from build123d import *

# Parameters (mm, degrees)
SKETCH2_R           = 1.5
BOSS_EXTRUDE1_DEPTH = 5


with BuildPart() as part:
    # Sketch2 → Boss-Extrude1 (new body)
    with BuildSketch(Plane.XY):
        with BuildLine():
            Line((5, -33), (5, -8.660254038))
            ThreePointArc((5, -8.660254038), (9.870667346, 1.603098918), (2.002269745, 9.797495388))
            Line((2.002269745, 9.797495388), (2.00266405, 11.49953636))
            Line((2.00266405, 11.49953636), (2.002664157, 11.499999691))
            ThreePointArc((2.002664157, 11.499999691), (0.002664157, 13.499999691), (-1.997335843, 11.499999691))
            Line((-1.997335843, 11.499999691), (-1.998003665, 8.617307095))
            ThreePointArc((-1.998003665, 8.617307095), (-3.567262635, 6.664705601), (-5.812270881, 7.776085051))
            Line((-5.812270881, 7.776085051), (-6.351761581, 8.938967191))
            ThreePointArc((-6.351761581, 8.938967191), (-9.315039529, 9.734283484), (-9.574251776, 6.677102885))
            Line((-9.574251776, 6.677102885), (-7.526953052, 4.647039677))
            ThreePointArc((-7.526953052, 4.647039677), (-7.244787999, 2.157941439), (-9.614515081, 1.345771067))
            Line((-9.614515081, 1.345771067), (-10.820227093, 1.781203427))
            ThreePointArc((-10.820227093, 1.781203427), (-13.469614339, 0.244947506), (-11.499566198, -2.099886252))
            Line((-11.499566198, -2.099886252), (-11.463831285, -2.099566981))
            Line((-11.463831285, -2.099566981), (-8.600020221, -2.073980428))
            ThreePointArc((-8.600020221, -2.073980428), (-6.633040893, -3.625608638), (-7.724488765, -5.880669462))
            Line((-7.724488765, -5.880669462), (-7.993660259, -6.008443697))
            Line((-7.993660259, -6.008443697), (-8.882563754, -6.430401321))
            ThreePointArc((-8.882563754, -6.430401321), (-9.651698384, -9.400582629), (-6.592349134, -9.632805038))
            Line((-6.592349134, -9.632805038), (-5.601479532, -8.615725566))
            ThreePointArc((-5.601479532, -8.615725566), (-5.218458324, -8.535632344), (-5, -8.860280046))
            Line((-5, -8.860280046), (-5, -33))
            ThreePointArc((-5, -33), (0, -38), (5, -33))
        make_face()
        with Locations((0, -33)):
            Circle(SKETCH2_R, mode=Mode.SUBTRACT)
        Circle(SKETCH2_R, mode=Mode.SUBTRACT)
    extrude(amount=BOSS_EXTRUDE1_DEPTH)


solid = part.part
Work out the finished part from the listing and answer in its coordinate system (mm). A direction names the side the tool comes from. Coordinates: 2 decimals unless noted, no trailing zeros. Loops run counter-clockwise (first coordinate to the right, second up) from the corner with the lowest first, then second, coordinate; pieces in that order, holes last. Notation, with made-up numbers: M 83.25,33 L 107.25,33 A14 ccw 107.25,44 Z; hole C 39,36.5 d7. An arc over 180 degrees is marked long. Answer in a Markdown table with one row per item. Add a question column.
1. The mould has two halves that part along X. Classify faces 1 (the cylindrical face through (0, -38, 2)), 2 (the cylindrical face through (-9.275, 9.762, 2.465)), 3 (the cylindrical face through (9.9, 1.4, 2.5)): pulls with the +X half, pulls with the -X half, needs draft (parallel to the pull), parting line crosses it, or undercut.
2. Find section B-B, the plane z = 2.95. State how many separate pieces and enclosed holes the cut face has, then the cut area to 3 significant figures.
3. Find section A-A, the plane x = 0. Write down the section's boundary in (y, z).
4. Consider L1, parallel to Y at x = 0, z = 3.2; L2, parallel to X at y = -10.5, z = 2.65; L3, parallel to X at y = 8.5, z = 0.45. Determine where each line is inside the solid, lowest interval first.
5. A tool of negligible diameter and unlimited length cuts with its end or side. For faces 4 (the flat face through (-6.08, 8.35, 2.46)), 5 (the flat face through (-8.565, 5.676, 2.465)), 6 (the flat face through (-10.21, 1.56, 2.46)), 7 (the flat face through (5, -21, 2)), 8 (the flat face through (-6.1, -9.13, 2.46)), from which of +Z, -Z, +X, -X, +Y, -Y can it reach the whole face along a straight path? Write none if from no direction.
6. Find section C-C, the plane y = 0. Write down the section's boundary in (x, z), then the cut area to 3 significant figures.
7. Find section D-D, the plane y = -22. Write down the section's boundary in (x, z), then the cut area to 3 significant figures.
8. Flat-ended cylindrical pins translate along their axes: P1, Ø1.5, axis at y = -21, z = 1.5, coming from the +X side; P2, Ø2.5, axis at y = 10, z = 3.5, coming from the -X side; P3, Ø1.5, axis at y = -21, z = 3.5, coming from the -X side. Find the tip coordinate at first contact, or state that the pin passes through.
Reported:
| question | item | result |
|---|---|---|
| 1 | face 1 | parting line crosses it |
| 1 | face 2 | undercut |
| 1 | face 3 | pulls with the +X half |
| 2 | separate pieces | 1 |
| 2 | enclosed holes | 2 |
| 2 | area | 598 mm^2 |
| 3 | outline | M -38,0 L -34.5,0 L -34.5,5 L -38,5 Z; M -31.5,0 L -1.5,0 L -1.5,5 L -31.5,5 Z; M 1.5,0 L 13.5,0 L 13.5,5 L 1.5,5 Z |
| 4 | L1 | y = -38 to -34.5, -31.5 to -1.5, 1.5 to 13.5 |
| 4 | L2 | x = -5 to 5 |
| 4 | L3 | x = -10.13 to -6.15, -2 to 5.27 |
| 5 | face 4 | +Z, -Z, +Y |
| 5 | face 5 | +Z, -Z, -X |
| 5 | face 6 | +Z, -Z |
| 5 | face 7 | +Z, -Z, +X, -Y |
| 5 | face 8 | +Z, -Z, -Y |
| 6 | outline | M -13.5,0 L -1.5,0 L -1.5,5 L -13.5,5 Z; M 1.5,0 L 10,0 L 10,5 L 1.5,5 Z |
| 6 | area | 102 mm^2 |
| 7 | outline | M -5,0 L 5,0 L 5,5 L -5,5 Z |
| 7 | area | 50.0 mm^2 |
| 8 | P1 | stops at x = 5 |
| 8 | P2 | stops at x = -10.06 |
| 8 | P3 | stops at x = -5 |
